from build123d import *

# Parameters (mm, degrees)
SKETCH1_W = 8
SKETCH1_H = 1
FILLET2_R = 0.2
FILLET3_R = 0.5


with BuildPart() as part:
    # Sketch1 → Revolve1 (revolve)
    with BuildSketch(Plane.XY, mode=Mode.PRIVATE) as revolve1_sk:
        with Locations((4, 3.5)):
            Rectangle(SKETCH1_W, SKETCH1_H)
    revolve(revolve1_sk.sketch.rotate(Axis((0, 0, 0), (1, 0, 0)), 90), axis=Axis((0, 0, 0), (1, 0, 0)))

    # Fillet2
    fillet2_edges = [part.edges().sort_by_distance(p)[0] for p in [
        (8, 0, -4),
        (0, 0, -4),
    ]]
    fillet(fillet2_edges, radius=FILLET2_R)

    # Fillet3
    fillet3_edges = [part.edges().sort_by_distance(p)[0] for p in [
        (8, 0, -3),
        (0, 0, -3),
    ]]
    fillet(fillet3_edges, radius=FILLET3_R)


solid = part.part
Design review of the part built by this model. Coordinates are the model's own, in mm. Give positions to 0.01 mm unless a question says otherwise; leave off trailing zeros. Loops run counter-clockwise (first coordinate to the right, second up) from the corner with the lowest first, then second, coordinate; pieces in that order, holes last. Notation, with made-up numbers: M 16,35.5 L 49,35.5 A14 cw 49,40.5 Z; hole C -25,-29.5 d4. An arc over 180 degrees is marked long. One line per question, with ' | ' between items. Start each with the question number.
1. Insertion check: P1, Ø4, axis at x = 3.5, y = -3, coming from the +Z side; P2, Ø2, axis at x = 1.5, y = 3, coming from the -Z side. Each pin has a flat end and moves straight along its axis. Give the tip position at first contact, or say it passes through.
2. To check wall thickness, follow L1, parallel to Y at x = 5.25, z = 0; L2, parallel to Y at x = 3.25, z = 2.75; L3, parallel to Z at x = 1.25, y = -1. State the ranges of each line that lie inside material, in increasing order.
3. Add section A-A (z = 0). Write out the cut boundary in (x, y), plus the area to 3 significant figures.
4. The part is to be moulded in two halves that separate along Y. For faces 1 (the face through (4.05, -0.9, 2.86)), 2 (the face through (4.053, 3.905, -0.867)), say which applies: released by +Y, released by -Y, zero draft, split by the parting line, or undercut.
5. Add section C-C (x = 2.25). Write out the cut boundary in (y, z), plus the area to 3 significant figures.
Worked out:
1) P1: stops at z = 3.87 | P2: stops at z = -3.46
2) L1: y = -4 to -3, 3 to 4 | L2: y = -2.9 to -1.2, 1.2 to 2.9 | L3: z = -3.87 to -2.83, 2.83 to 3.87
3) outline: M 0,-3.8 A0.2 ccw 0.2,-4 L 7.8,-4 A0.2 ccw 8,-3.8 L 8,-3.5 A0.5 ccw 7.5,-3 L 0.5,-3 A0.5 ccw 0,-3.5 Z; M 0,3.5 A0.5 ccw 0.5,3 L 7.5,3 A0.5 ccw 8,3.5 L 8,3.8 A0.2 ccw 7.8,4 L 0.2,4 A0.2 ccw 0,3.8 Z | area: 15.8 mm²
4) face 1: undercut | face 2: split by the parting line
5) outline: C 0,0 d8; hole C 0,0 d6 | area: 22.0 mm²
